Geometry: final body of the model. Coordinates: model frame, mm. Face numbers are marked on the shaded views. A direction names the side the tool comes from. Give positions to 0.01 mm unless a question says otherwise; leave off trailing zeros. Loops run counter-clockwise (first coordinate to the right, second up) from the corner with the lowest first, then second, coordinate; pieces in that order, holes last. Notation, with made-up numbers: (57, -5) -> (108, -5) arc R25 ccw to (108, 27) -> close; hole circle Ø5 at (-17.5, 73.25). An arc over 180 degrees is marked (long way). One line per question, with ' | ' between items. Start each with the question number.
Item 1: Pin query (flat end, axial travel): P1, Ø12, axis at x = -9.5, y = 27.5, coming from the -Z side; P2, Ø3, axis at x = -17, z = 4, coming from the +Y side; P3, Ø6, axis at y = 23.5, z = 2.5, coming from the -X side. Return the tip coordinate at first contact, or that it passes through.
Item 2: Material intervals for line 1 along Y through (x, z) = (-17.75, 6.35); line 2 along Y through (x, z) = (-20, 0.75), sorted ascending. Write a range as [from, to].
Item 3: Section B-B on z = 6.35. Return loops of the section in (x, y) (3 decimals), then the cut area to 3 significant figures.
Item 4: Set-up query: the marked faces 1 and 2. Return all of +Z, -Z, +X, -X, +Y, -Y with unobstructed straight access to the full face (end or side cutting, diameter ignored); none if empty.
Item 5: Section D-D on z = 10.5. Return loops of the section in (x, y) (3 decimals), then the cut area to 3 significant figures.
Item 6: Section A-A on x = -11.5. Return loops of the section in (y, z), then the cut area to 3 significant figures.
Item 7: Mould query, pull axis Z, two halves, no side actions, for the marked faces 3, 4 and 5. Classes: released by +Z, released by -Z, zero draft, split by the parting line, or undercut.
Item 8: Section C-C on x = -5.5. Return loops of the section in (y, z).
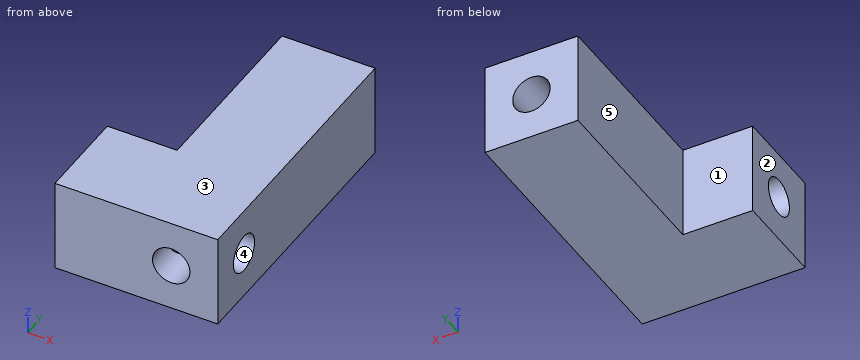
from build123d import *

# Parameters (mm, degrees)
BOSS_EXTRUDE1_DEPTH     = 12.7
F_1_4_20_TAPPED_HOLE1_D = 5.1054
F_1_4_20_TAPPED_HOLE2_D = 5.1054


with BuildPart() as part:
    # Sketch1 → Boss-Extrude1 (new body)
    with BuildSketch(Plane.XY):
        Polygon((0, 0), (0, 38.1), (-12.7, 38.1), (-12.7, 12.7), (-22.225, 12.7), (-22.225, 0), align=None)
    extrude(amount=BOSS_EXTRUDE1_DEPTH)

    # 1/4-20 Tapped Hole1 (through all)
    with Locations(Plane(origin=(0, 38.1, 0), x_dir=(1, 0, 0), z_dir=(0, 1, 0))):
        with Locations((-6.35, -6.35)):
            Hole(F_1_4_20_TAPPED_HOLE1_D / 2)

    # 1/4-20 Tapped Hole2 (through all)
    with Locations(Plane.ZY.offset(22.225)):
        with Locations((6.35, 6.35)):
            Hole(F_1_4_20_TAPPED_HOLE2_D / 2)


solid = part.part
Result sheet:
1) P1: stops at z = 0 | P2: stops at y = 12.7 | P3: stops at x = -12.7
2) line 1: y = [0, 3.8], [8.9, 12.7] | line 2: y = [0, 12.7]
3) outline: (-22.225, 0) -> (-8.903, 0) -> (-8.903, 3.797) -> (-22.225, 3.797) -> close; (-22.225, 8.903) -> (-8.903, 8.903) -> (-8.903, 38.1) -> (-12.7, 38.1) -> (-12.7, 12.7) -> (-22.225, 12.7) -> close; (-3.797, 0) -> (0, 0) -> (0, 3.797) -> (-3.797, 3.797) -> close; (-3.797, 8.903) -> (0, 8.903) -> (0, 38.1) -> (-3.797, 38.1) -> close | area: 323 mm²
4) face 1: +Z, -Z, -X, +Y | face 2: +Z, -Z, -X, +Y, -Y
5) outline: (-22.225, 0) -> (0, 0) -> (0, 38.1) -> (-12.7, 38.1) -> (-12.7, 12.7) -> (-22.225, 12.7) -> close | area: 605 mm²
6) outline: (0, 0) -> (38.1, 0) -> (38.1, 12.7) -> (0, 12.7) -> close; hole circle Ø5.11 at (6.35, 6.35) | area: 463 mm²
7) face 3: released by +Z | face 4: undercut | face 5: zero draft
8) outline: (0, 0) -> (38.1, 0) -> (38.1, 3.94) -> (7.2, 3.94) arc R2.55 cw to (5.5, 3.94) -> (0, 3.94) -> close; (0, 8.76) -> (5.5, 8.76) arc R2.55 cw to (7.2, 8.76) -> (38.1, 8.76) -> (38.1, 12.7) -> (0, 12.7) -> close
